Part model, mm, in its own coordinate system. Give positions to 0.01 mm unless a question says otherwise; leave off trailing zeros. Write each loop counter-clockwise with the first axis right and the second up, starting at its lowest first coordinate (ties: lowest second). Pieces come first, ordered by that corner, then holes. Notation, with made-up numbers: M -24,77 L 11,77 A7 cw 11,81 Z; hole C 51.5,33.25 d3. An arc over 180 degrees is marked long. Answer as CSV lines item,"result". Start each with the question number.
1) Wall check: line 1 along X through (y, z) = (20.5, 3.75); line 2 along Y through (x, z) = (109, 1.9); line 3 along X through (y, z) = (118.5, 1.65). Give the ranges that are in metal, low to high. Write a range as from..to.
2) Slice it at A-A, the plane x = 95.5. Give the cut face in (y, z), plus the area to 3 significant figures.
3) Slice it at B-B, the plane z = 1.3. Give the cut face in (x, y), plus the area to 3 significant figures.
```python
from build123d import *

# Parameters (mm, degrees)
MODEL_W             = 150
MODEL_H             = 120
MODEL_R             = 1.5
BOSS_EXTRUDE1_DEPTH = 5
CUT_EXTRUDE1_DEPTH  = 207.889226408


with BuildPart() as part:
    # Model → Boss-Extrude1 (new body)
    with BuildSketch(Plane.XY):
        with Locations((86.555612284, 69.143083993)):
            Rectangle(MODEL_W, MODEL_H)
        with Locations((22.178986017, 117.822854057)):
            Circle(MODEL_R, mode=Mode.SUBTRACT)
        with Locations((150.932238551, 117.822854057)):
            Circle(MODEL_R, mode=Mode.SUBTRACT)
        with Locations((22.178986017, 20.46331393)):
            Circle(MODEL_R, mode=Mode.SUBTRACT)
        with Locations((150.932238551, 20.46331393)):
            Circle(MODEL_R, mode=Mode.SUBTRACT)
    extrude(amount=BOSS_EXTRUDE1_DEPTH)

    # Sketch2 → Cut-Extrude1 (cut, through all)
    with BuildSketch(Plane.XY.offset(5)):
        with BuildLine():
            Line((56.551143806, 115.585597336), (116.559939574, 115.69114655))
            ThreePointArc((116.559939574, 115.69114655), (119.104909718, 113.155113361), (116.568876529, 110.610143217))
            Line((116.568876529, 110.610143217), (56.560080761, 110.504594003))
            ThreePointArc((56.560080761, 110.504594003), (54.015110617, 113.040627192), (56.551143806, 115.585597336))
        make_face()
        with BuildLine():
            Line((56.560484104, 28.010889901), (116.569279872, 27.905340687))
            ThreePointArc((116.569279872, 27.905340687), (119.334225635, 25.130651283), (116.559536231, 22.36570552))
            Line((116.559536231, 22.36570552), (56.550740464, 22.471254734))
            ThreePointArc((56.550740464, 22.471254734), (53.7857947, 25.245944138), (56.560484104, 28.010889901))
        make_face()
    extrude(amount=-CUT_EXTRUDE1_DEPTH, mode=Mode.SUBTRACT)


solid = part.part
```
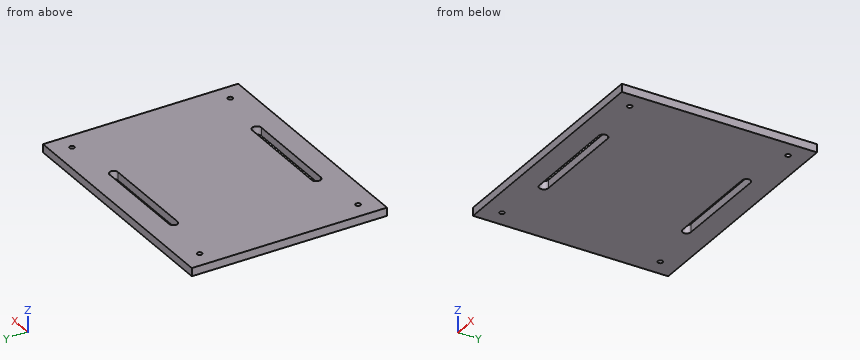
Found:
1,line 1,"11.56..20.68, 23.68..149.43, 152.43..161.56"
1,line 2,"9.14..22.38, 27.92..110.6, 115.68..129.14"
1,line 3,"11.56..20.84, 23.52..149.59, 152.27..161.56"
2,outline,"M 9.14,0 L 22.4,0 L 22.4,5 L 9.14,5 Z; M 27.94,0 L 110.57,0 L 110.57,5 L 27.94,5 Z; M 115.65,0 L 129.14,0 L 129.14,5 L 115.65,5 Z"
2,area,"547 mm²"
3,outline,"M 11.56,9.14 L 161.56,9.14 L 161.56,129.14 L 11.56,129.14 Z; hole C 22.18,20.46 d3; hole C 22.18,117.82 d3; hole M 56.55,22.47 L 116.56,22.37 A2.77 ccw 116.57,27.91 L 56.56,28.01 A2.77 ccw Z; hole M 56.55,115.59 A2.54 ccw 56.56,110.5 L 116.57,110.61 A2.54 ccw 116.56,115.69 Z; hole C 150.93,20.46 d3; hole C 150.93,117.82 d3"
3,area,"17,300 mm²"
